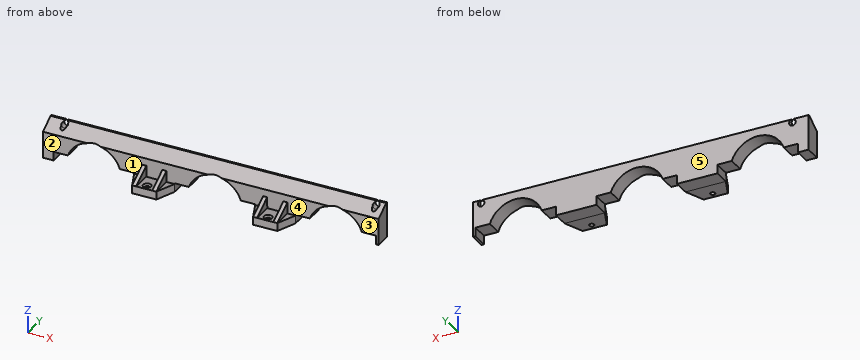
```python
from build123d import *

# Parameters (mm, degrees)
BOSS_EXTRUDE3_DEPTH        = 10
SKETCH4_R                  = 1.5
BOSS_EXTRUDE4_DEPTH        = 5
RIB6_REACH                 = 158.985
SKETCH5_WALL_W             = 329.861950248
SKETCH5_WALL_H             = 2.5
CHAMFER2_SIZE              = 1
CHAMFER3_SIZE              = 5.5
CHAMFER3_SIZE_2            = 9
LPATTERN4_COUNT            = 2
LPATTERN4_PITCH            = 75
LPATTERN4_COPY_1_REACH     = 158.985
LPATTERN4_COPY_1_SKETCH_W  = 329.861950248
LPATTERN4_COPY_1_SKETCH_H  = 2.5
CHAMFER2_OF_LPATTERN4_SIZE = 1
SKETCH8_R                  = 2.05
CUT_EXTRUDE1_DEPTH         = 4
SKETCH9_R                  = 1.6
CUT_EXTRUDE2_DEPTH         = 5
SZKIC1_W                   = 8.551960468
SZKIC1_H                   = 23.590081372
WYTNIJ_WYCI_GNI_CIE3_DEPTH = 30.5


with BuildPart() as part:
    # Sketch2 → Boss-Extrude3 (new body)
    with BuildSketch(Plane(origin=(0, 0, 0), x_dir=(1, 0, 0), z_dir=(0, 1, 0))):
        with BuildLine():
            Line((-138.973021921, 39.179223473), (-139.022764358, 17.179279707))
            Line((-139.022764358, 17.179279707), (73.976691191, 16.697682479))
            Line((73.976691191, 16.697682479), (74.026978079, 38.697625014))
            Line((74.026978079, 38.697625014), (67.526578048, 38.712322585))
            Line((67.526578048, 38.712322585), (67.51414235, 33.212297518))
            Line((67.51414235, 33.212297518), (58.599731895, 33.232453229))
            ThreePointArc((58.599731895, 33.232453229), (42.488076808, 21.768891824), (26.428425, 33.305193378))
            Line((26.428425, 33.305193378), (17.51414235, 33.3253488))
            Line((17.51414235, 33.3253488), (17.526578048, 38.825373866))
            Line((17.526578048, 38.825373866), (-7.473230244, 38.881899074))
            Line((-7.473230244, 38.881899074), (-7.485665941, 33.381874007))
            Line((-7.485665941, 33.381874007), (-16.400076396, 33.402029717))
            ThreePointArc((-16.400076396, 33.402029717), (-32.511731484, 21.938468313), (-48.571383292, 33.474769867))
            Line((-48.571383292, 33.474769867), (-57.485665941, 33.494925288))
            Line((-57.485665941, 33.494925288), (-57.473230244, 38.994950355))
            Line((-57.473230244, 38.994950355), (-82.473038536, 39.051475562))
            Line((-82.473038536, 39.051475562), (-82.485474233, 33.551450496))
            Line((-82.485474233, 33.551450496), (-91.399884688, 33.571606206))
            ThreePointArc((-91.399884688, 33.571606206), (-107.511539776, 22.108044802), (-123.571191584, 33.644346356))
            Line((-123.571191584, 33.644346356), (-132.485474233, 33.664501777))
            Line((-132.485474233, 33.664501777), (-132.473038536, 39.164526844))
            Line((-132.473038536, 39.164526844), (-138.973021921, 39.179223473))
        make_face()
    extrude(amount=BOSS_EXTRUDE3_DEPTH)

    # Sketch4 → Boss-Extrude4 (add)
    with BuildSketch(Plane(origin=(0.087874316, 0, -38.864803222), x_dir=(-0.99999744389135, 0, -0.002261019850970016), z_dir=(0.002261019850970016, 0, -0.99999744389135))):
        Polygon((62.56118779, -12), (57.561251693, 0), (82.561123887, 0), (77.56118779, -12), align=None)
        with Locations((70.06118779, -8.5)):
            Circle(SKETCH4_R, mode=Mode.SUBTRACT)
    boss_extrude4 = extrude(amount=-BOSS_EXTRUDE4_DEPTH)

    # Sketch5 wall → Rib6 (add, up to next)
    with BuildSketch(Plane(origin=(-77.492333887, -6, -30.540192335), x_dir=(-0.001139262394, 0.863778900906, 0.503869737562), z_dir=(-0.001953021242, -0.503871025511, 0.863776692993)), mode=Mode.PRIVATE) as rib6_sk1:
        with Locations((0, -1.25)):
            Rectangle(SKETCH5_WALL_W, SKETCH5_WALL_H)
    rib6_tool1 = extrude(rib6_sk1.sketch, amount=-RIB6_REACH, mode=Mode.PRIVATE) - part.part
    rib6 = rib6_tool1.solids().sort_by_distance((-77.492333887, -6, -30.540192335))[0]
    add(rib6)

    # Mirror2: Rib6 across plane
    add(rib6.mirror(Plane(origin=(-70.061008706, 0, -0.158409736), x_dir=(-0.0022610198509701073, 0, 0.99999744389135), z_dir=(0.99999744389135, 0, 0.002261019850970107))))

    # Chamfer2
    chamfer2_edges = [part.edges().sort_by_distance(p)[0] for p in [
        (-68.484443323, -8.5, -34.01983421),
    ]]
    chamfer(chamfer2_edges, length=CHAMFER2_SIZE)

    # Chamfer3
    # the kernel refuses this chamfer: 9, 5.5 mm, written as the material it takes off along each edge
    with BuildSketch(Plane(origin=(-162.295390883, 0, -17.231899712), x_dir=(0.0022577295255832275, -0.053929224624231706, -0.9985422081158205), z_dir=(0.9999974438913499, 0, 0.0022610198509699707))) as chamfer3_piece_1:
        Polygon((CHAMFER3_SIZE * 0.998544760505, CHAMFER3_SIZE * 0.0539292246242), (-CHAMFER3_SIZE_2 * 0.0539292246242, CHAMFER3_SIZE_2 * 0.998544760505), (0, 0), align=None)
    extrude(amount=259.545372026, mode=Mode.SUBTRACT)

    # LPattern4: Boss-Extrude4, Rib6 ×2
    with Locations(*[Vector(0.9999974438913499, 0, 0.0022610198509701) * (i * LPATTERN4_PITCH) for i in range(1, LPATTERN4_COUNT)]):
        add(boss_extrude4)
        add(rib6)

    # LPattern4 copy 1 sketch → LPattern4 copy 1 (add, up to next)
    with BuildSketch(Plane(origin=(12.507436062, -6, -30.336700548), x_dir=(-0.0011392623880184954, 0.863778900906, 0.5038697375620136), z_dir=(-0.0019530212415939509, -0.503871025511, 0.863776692993001)), mode=Mode.PRIVATE) as lpattern4_copy_1_sk1:
        with Locations((0, 1.25)):
            Rectangle(LPATTERN4_COPY_1_SKETCH_W, LPATTERN4_COPY_1_SKETCH_H)
    lpattern4_copy_1_tool1 = extrude(lpattern4_copy_1_sk1.sketch, amount=-LPATTERN4_COPY_1_REACH, mode=Mode.PRIVATE) - part.part
    add(lpattern4_copy_1_tool1.solids().sort_by_distance((12.507436062, -6, -30.336700548))[0])

    # Chamfer2 of LPattern4
    chamfer2_of_lpattern4_edges = [part.edges().sort_by_distance(p)[0] for p in [
        (6.515364969, -8.5, -33.850257721),
    ]]
    chamfer(chamfer2_of_lpattern4_edges, length=CHAMFER2_OF_LPATTERN4_SIZE)

    # Sketch8 → Cut-Extrude1 (cut)
    with BuildSketch(Plane(origin=(0, 10, 0), x_dir=(1, 0, 0), z_dir=(0, 1, 0))):
        with Locations((-129.018242433, 19.156613217)):
            Circle(SKETCH8_R)
    cut_extrude1 = extrude(amount=-CUT_EXTRUDE1_DEPTH, mode=Mode.SUBTRACT)

    # Sketch9 → Cut-Extrude2 (cut)
    with BuildSketch(Plane(origin=(0, 6, 0), x_dir=(1, 0, 0), z_dir=(0, 1, 0))):
        with Locations((-129.018242433, 19.156613217)):
            Circle(SKETCH9_R)
    cut_extrude2 = extrude(amount=-CUT_EXTRUDE2_DEPTH, mode=Mode.SUBTRACT)

    # Mirror4: Cut-Extrude1, Cut-Extrude2 across plane
    add(cut_extrude1.mirror(Plane(origin=(-32.561168463, 0, -0.073621636), x_dir=(-0.002261019850969509, 0, 0.99999744389135), z_dir=(-0.99999744389135, 0, -0.0022610198509695084))), mode=Mode.SUBTRACT)
    add(cut_extrude2.mirror(Plane(origin=(-32.561168463, 0, -0.073621636), x_dir=(-0.002261019850969509, 0, 0.99999744389135), z_dir=(-0.99999744389135, 0, -0.0022610198509695084))), mode=Mode.SUBTRACT)

    # Szkic1 → Wytnij-wyciągnięcie3 (cut)
    with BuildSketch(Plane(origin=(0, 10, 0), x_dir=(1, 0, 0), z_dir=(0, 1, 0))):
        with Locations((73.302426643, 26.913890658)):
            Rectangle(SZKIC1_W, SZKIC1_H)
    extrude(amount=-WYTNIJ_WYCI_GNI_CIE3_DEPTH, mode=Mode.SUBTRACT)


solid = part.part
```
Source: CAD feature listing. Evaluate the final solid. Frame: model axes, mm. Face numbers are marked on the shaded views. A direction names the side the tool comes from. Coordinates: 2 decimals unless noted, no trailing zeros. Write each loop counter-clockwise with the first axis right and the second up, starting at its lowest first coordinate (ties: lowest second). Pieces come first, ordered by that corner, then holes. Notation, with made-up numbers: (70, 6.25) - (91, 6.25) arc R18 cw to (91, 15.25) - close; hole circle Ø9 at (-40, 50). An arc over 180 degrees is marked (long way). Answer as a JSON object with one key per item and string values.
Q1. Material intervals for line 1 (X direction, y = -3.75, z = -33.25); line 2 (X direction, y = 1, z = -37.75); line 3 (Y direction, x = -122.5, z = -29.75), sorted ascending. Write a range as [from, to].
Ans:
{"line 1": "x = [-77.49, -74.99], [-64.99, -62.49], [-2.49, 0.01], [10.01, 12.51]", "line 2": "x = [-138.98, -132.48], [-82.48, -57.48], [-7.48, 17.52], [67.52, 69.03]", "line 3": "y = [0, 10]"}
Q2. Set-up query: the marked faces 3, 4 and 5. Return all of +Z, -Z, +X, -X, +Y, -Y with unobstructed straight access to the full face (end or side cutting, diameter ignored); none if empty.
Ans:
{"face 3": "+Z, -Z, +X, -Y", "face 4": "+Z, -Y", "face 5": "+Z, -Z, +X, -X, +Y"}
Q3. Section query B-B, the plane x = 14.5. Output: boundary loops of the cut face in (y, z), plus the area to 3 significant figures.
Ans:
{"outline": "(-7.26, -38.83) - (10, -38.83) - (10, -16.83) - (9, -16.83) - (0, -22.33) - (0, -33.83) - (-7.24, -33.83) - close", "area": "232 mm2"}
Q4. Section query D-D, the plane x = -13. Output: boundary loops of the cut face in (y, z), plus the area to 3 significant figures.
Ans:
{"outline": "(0, -33.39) - (10, -33.39) - (10, -16.89) - (9, -16.89) - (0, -22.39) - close", "area": "140 mm2"}
Q5. First-contact query: pin 1 Ø3.5 at (x, z) = (-54, -31) entering from -Y; pin 2 Ø3 at (y, z) = (-8.5, -30.5) entering from -X; pin 3 Ø2.5 at (x, z) = (-128.5, -19.5) entering from +Y; pin 4 Ø2.5 at (x, z) = (64, -20) entering from +Y. Flat tips, straight axial feed; report the tip coordinate or a pass-through.
Ans:
{"pin 1": "stops at y = 0", "pin 2": "stops at x = -77.49", "pin 3": "stops at y = 6", "pin 4": "stops at y = 10"}
Q6. Draft query along X for the marked faces 1 and 2. Return one class per face: released by +X, released by -X, zero draft, split by the parting line, or undercut.
Ans:
{"face 1": "undercut", "face 2": "zero draft"}
Q7. Section query A-A, the plane y = -3. Output: boundary loops of the cut face in (x, z).
Ans:
{"outline": "(-81.23, -34.05) - (-81.22, -39.05) - (-58.72, -39) - (-58.73, -34) - (-62.48, -34.01) - (-62.5, -28.76) - (-65, -28.76) - (-64.98, -34.01) - (-74.98, -34.03) - (-75, -28.78) - (-77.5, -28.79) - (-77.48, -34.04) - close; (-6.23, -33.88) - (-6.22, -38.88) - (16.28, -38.83) - (16.27, -33.83) - (12.52, -33.84) - (12.5, -28.59) - (10, -28.59) - (10.02, -33.84) - (0.02, -33.86) - (0, -28.61) - (-2.5, -28.62) - (-2.48, -33.87) - close"}
Q8. Section query C-C, the plane z = -37. State how many separate pieces and enclosed holes the cut face has, plus the area to 3 significant figures.
Ans:
{"separate pieces": "4", "enclosed holes": "2", "area": "1,050 mm2"}
